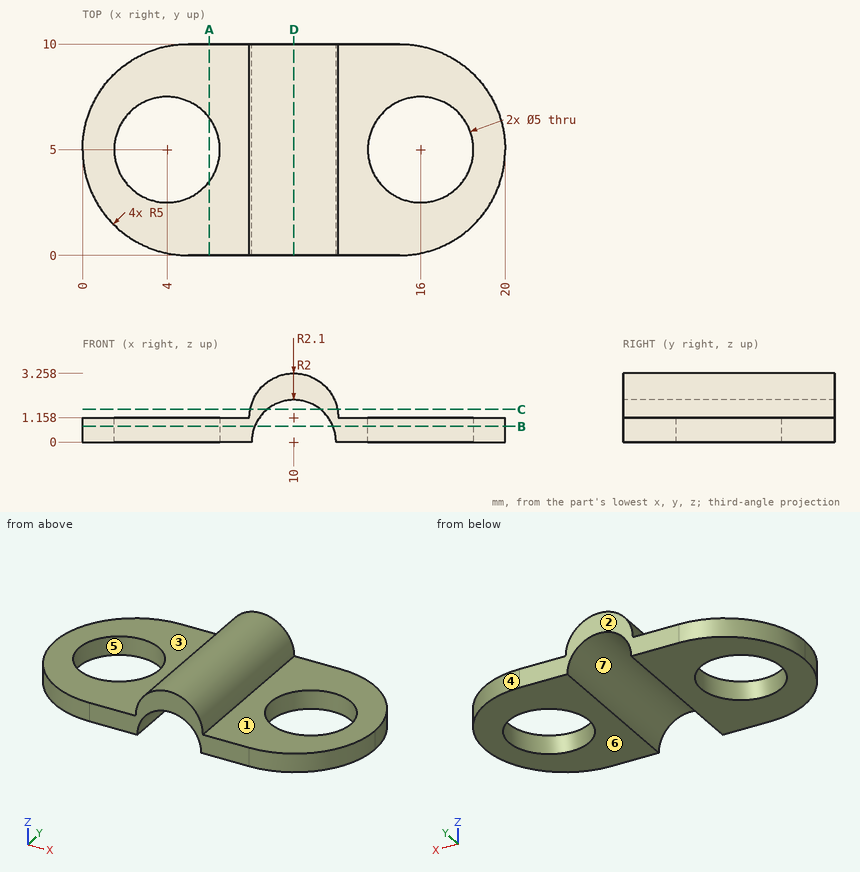
Job drawing, mm, ordinate dimensions from the low corner. One solid piece. A direction names the side the tool comes from. Coordinates: 2 decimals unless noted, no trailing zeros. Write each loop counter-clockwise with the first axis right and the second up, starting at its lowest first coordinate (ties: lowest second). Pieces come first, ordered by that corner, then holes. Notation, with made-up numbers: (-8.5, -17.75) - (17.5, -17.75) arc R25 ccw to (17.5, 1.25) - close; hole circle Ø10 at (-13.5, 52). An arc over 180 degrees is marked (long way). Use a Markdown table: item, result. Add a question column.
Item 1: Band-saw the part on D-D, the plane x = 10. Give the cut face in (y, z), and give its area (3 significant figures).
Item 2: Flat gauge pins, fed straight in: pin 1 (1 mm diameter, centred on y = 3.5, z = 1.5, fed in from +X); pin 2 (6 mm diameter, centred on x = 4, y = 5, fed in from +Z); pin 3 (1.5 mm diameter, centred on x = 2.5, y = 4, fed in from -Z); pin 4 (1.5 mm diameter, centred on y = 6.5, z = 2, fed in from -X). Where does each tip first touch, or does it go through?
Item 3: Band-saw the part on B-B, the plane z = 0.75. Give the number of separate pieces and of enclosed holes in the cut face, and give its area (3 significant figures).
Item 4: 3-axis set-ups, long thin cutter, end or side, ignore diameter. For the marked faces 1, 2 and 3: which of +Z, -Z, +X, -X, +Y, -Y reach the whole face in a straight line?
Item 5: Band-saw the part on C-C, the plane z = 1.55. Give the cut face in (x, y), and give its area (3 significant figures).
Item 6: Mould opens along X. For the marked faces 4, 5, 6 and 7 say: pulls with the +X half, pulls with the -X half, needs draft (parallel to the pull), parting line crosses it, or undercut.
Item 7: Band-saw the part on A-A, the plane x = 6. Give the cut face in (y, z).
Item 8: Drill centre lines: L1, parallel to X at y = 3.5, z = 0.7; L2, parallel to Z at x = 6, y = 7.5; L3, parallel to Y at x = 4, z = 0.45. Where is each one in solid material? Low to high. Write a range as from..to.
Numbers:
| question | item | result |
|---|---|---|
| 1 | outline | (0, 2) - (10, 2) - (10, 3.26) - (0, 3.26) - close |
| 1 | area | 12.6 mm2 |
| 2 | pin 1 | x = 19.87 |
| 2 | pin 2 | z = 1.16 |
| 2 | pin 3 | z = 0 |
| 2 | pin 4 | x = 7.9 |
| 3 | separate pieces | 2 |
| 3 | enclosed holes | 2 |
| 3 | area | 102 mm2 |
| 4 | face 1 | +Z, +X, +Y, -Y |
| 4 | face 2 | +Z, -Z, +X, -X, +Y |
| 4 | face 3 | +Z, -X, +Y, -Y |
| 5 | outline | (7.94, 0) - (8.74, 0) - (8.74, 10) - (7.94, 10) - close; (11.26, 0) - (12.06, 0) - (12.06, 10) - (11.26, 10) - close |
| 5 | area | 16.0 mm2 |
| 6 | face 4 | pulls with the +X half |
| 6 | face 5 | undercut |
| 6 | face 6 | needs draft |
| 6 | face 7 | undercut |
| 7 | outline | (0, 0) - (3.5, 0) - (3.5, 1.16) - (0, 1.16) - close; (6.5, 0) - (10, 0) - (10, 1.16) - (6.5, 1.16) - close |
| 8 | L1 | 0.23..2, 6..8.13, 11.87..14, 18..19.77 |
| 8 | L2 | 0..1.16 |
| 8 | L3 | 0.1..2.5, 7.5..9.9 |
